CAD build for the part. Positions are in the model's coordinates, mm. Face numbers are marked on the shaded views. A direction names the side the tool comes from. Give positions to 0.01 mm unless a question says otherwise; leave off trailing zeros. Write each loop counter-clockwise with the first axis right and the second up, starting at its lowest first coordinate (ties: lowest second). Pieces come first, ordered by that corner, then holes. Notation, with made-up numbers: (-8, 62.25) -> (9, 62.25) arc R23 ccw to (9, 86.25) -> close; hole circle Ø8 at (17.25, 83). An arc over 180 degrees is marked (long way). Answer as a JSON object with one key per item and string values.
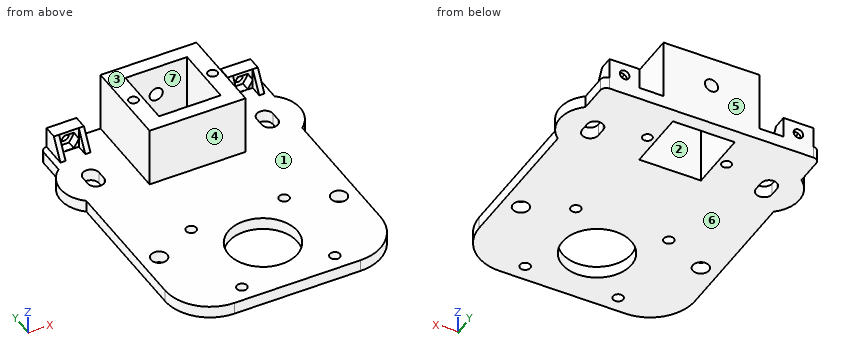
```python
from build123d import *

# Parameters (mm, degrees)
SKETCH_1_R          = 1.7
SKETCH_1_R_2        = 11.5
SKETCH_1_R_3        = 2.7
SKETCH_1_R_4        = 1.6
SKETCH_1_W          = 20.6
SKETCH_1_H          = 20.6
EXTRUDE_1_DEPTH     = 4
EXTRUDE_START       = 4
SKETCH_1_3_W        = 10
SKETCH_1_3_H        = 4.5
EXTRUDE_2_DEPTH     = 7
SKETCH_1_4_W        = 32
SKETCH_1_4_H        = 30
SKETCH_1_4_R        = 1.6
SKETCH_1_4_W_2      = 20.6
SKETCH_1_4_H_2      = 20.6
EXTRUDE_3_DEPTH     = 20
RIB_1_REACH         = 94.748
SKETCH_3_WALL_W     = 195.558888446
SKETCH_3_WALL_H     = 1.7
RIB_2_REACH         = 86.984
SKETCH_4_WALL_W     = 180.029901728
SKETCH_4_WALL_H     = 1.7
CUT_EXTRUDE_1_REACH = 104.259
SKETCH_5_R          = 2.2
SKETCH_5_R_2        = 1.6
CUT_EXTRUDE_2_DEPTH = 3


with BuildPart() as part:
    # 草图1 → 凸台-拉伸1 (new body)
    with BuildSketch(Plane.XY):
        with BuildLine():
            ThreePointArc((36, 48.5), (35.414213562, 49.914213562), (34, 50.5))
            Line((34, 50.5), (-34, 50.5))
            ThreePointArc((-34, 50.5), (-35.414213562, 49.914213562), (-36, 48.5))
            Line((-36, 48.5), (-36, 39.485281374))
            ThreePointArc((-36, 39.485281374), (-40, 31), (-36, 22.514718626))
            Line((-36, 22.514718626), (-36, -25.5))
            ThreePointArc((-36, -25.5), (-31.606601718, -36.106601718), (-21, -40.5))
            Line((-21, -40.5), (21, -40.5))
            ThreePointArc((21, -40.5), (31.606601718, -36.106601718), (36, -25.5))
            Line((36, -25.5), (36, 22.514718626))
            ThreePointArc((36, 22.514718626), (40, 31), (36, 39.485281374))
            Line((36, 39.485281374), (36, 48.5))
        make_face()
        with Locations((-15.5, -35)):
            Circle(SKETCH_1_R, mode=Mode.SUBTRACT)
        with Locations((15.5, -35)):
            Circle(SKETCH_1_R, mode=Mode.SUBTRACT)
        with Locations((0, -19.5)):
            Circle(SKETCH_1_R_2, mode=Mode.SUBTRACT)
        with Locations((-30, -11)):
            Circle(SKETCH_1_R_3, mode=Mode.SUBTRACT)
        with Locations((-15.5, -4)):
            Circle(SKETCH_1_R, mode=Mode.SUBTRACT)
        with Locations((30, -11)):
            Circle(SKETCH_1_R_3, mode=Mode.SUBTRACT)
        with Locations((15.5, -4)):
            Circle(SKETCH_1_R, mode=Mode.SUBTRACT)
        with BuildLine():
            Line((-26.3, 32.5), (-26.3, 29.5))
            ThreePointArc((-26.3, 29.5), (-29, 26.8), (-31.7, 29.5))
            Line((-31.7, 29.5), (-31.7, 32.5))
            ThreePointArc((-31.7, 32.5), (-29, 35.2), (-26.3, 32.5))
        make_face(mode=Mode.SUBTRACT)
        with BuildLine():
            Line((31.7, 32.5), (31.7, 29.5))
            ThreePointArc((31.7, 29.5), (29, 26.8), (26.3, 29.5))
            Line((26.3, 29.5), (26.3, 32.5))
            ThreePointArc((26.3, 32.5), (29, 35.2), (31.7, 32.5))
        make_face(mode=Mode.SUBTRACT)
        with Locations((13.2, 35.5)):
            Circle(SKETCH_1_R_4, mode=Mode.SUBTRACT)
        with Locations((0, 35.5)):
            Rectangle(SKETCH_1_W, SKETCH_1_H, mode=Mode.SUBTRACT)
        with Locations((-13.2, 35.5)):
            Circle(SKETCH_1_R_4, mode=Mode.SUBTRACT)
    extrude(amount=EXTRUDE_1_DEPTH)

    # 草图1<3> → 凸台-拉伸2 (add)
    with BuildSketch(Plane.XY.offset(EXTRUDE_START)):
        with Locations((-29, 48.25)):
            Rectangle(SKETCH_1_3_W, SKETCH_1_3_H)
        with Locations((29, 48.25)):
            Rectangle(SKETCH_1_3_W, SKETCH_1_3_H)
    extrude(amount=EXTRUDE_2_DEPTH)

    # 草图1<4> → 凸台-拉伸3 (add)
    with BuildSketch(Plane.XY.offset(EXTRUDE_START)):
        with Locations((0, 35.5)):
            Rectangle(SKETCH_1_4_W, SKETCH_1_4_H)
        with Locations((-13.2, 35.5)):
            Circle(SKETCH_1_4_R, mode=Mode.SUBTRACT)
        with Locations((0, 35.5)):
            Rectangle(SKETCH_1_4_W_2, SKETCH_1_4_H_2, mode=Mode.SUBTRACT)
        with Locations((13.2, 35.5)):
            Circle(SKETCH_1_4_R, mode=Mode.SUBTRACT)
    extrude(amount=EXTRUDE_3_DEPTH)

    # 草图3 wall → 筋1 (add, up to next)
    with BuildSketch(Plane(origin=(-34, 44, 7.5), x_dir=(0, -0.496138938357, -0.868243142124), z_dir=(0, -0.868243142124, 0.496138938357)), mode=Mode.PRIVATE) as rib_1_sk1:
        with Locations((0, 0.85)):
            Rectangle(SKETCH_3_WALL_W, SKETCH_3_WALL_H)
    rib_1_tool1 = extrude(rib_1_sk1.sketch, amount=-RIB_1_REACH, mode=Mode.PRIVATE) - part.part
    rib_1 = rib_1_tool1.solids().sort_by_distance((-34, 44, 7.5))[0]
    add(rib_1)

    # 草图4 wall → 筋2 (add, up to next)
    with BuildSketch(Plane(origin=(-24, 44, 7.5), x_dir=(0, -0.496138938357, -0.868243142124), z_dir=(0, 0.868243142124, -0.496138938357)), mode=Mode.PRIVATE) as rib_2_sk1:
        with Locations((0, 0.85)):
            Rectangle(SKETCH_4_WALL_W, SKETCH_4_WALL_H)
    rib_2_tool1 = extrude(rib_2_sk1.sketch, amount=RIB_2_REACH, mode=Mode.PRIVATE) - part.part
    rib_2 = rib_2_tool1.solids().sort_by_distance((-24, 44, 7.5))[0]
    add(rib_2)

    # 镜向1: 筋1, 筋2 across plane
    add(rib_1.mirror(Plane(origin=(0, 0, 0), x_dir=(0, 0, 1), z_dir=(1, 0, 0))))
    add(rib_2.mirror(Plane(origin=(0, 0, 0), x_dir=(0, 0, 1), z_dir=(1, 0, 0))))

    # 草图5 → 切除-拉伸1 (cut, up to next)
    with BuildSketch(Plane(origin=(0, 50.5, 0), x_dir=(1, 0, 0), z_dir=(0, 1, 0)), mode=Mode.PRIVATE) as cut_extrude_1_sk1:
        with Locations(Location((0, -14, 0), (0, 0, 270))):
            Circle(SKETCH_5_R)
    cut_extrude_1_tool1 = extrude(cut_extrude_1_sk1.sketch, amount=-CUT_EXTRUDE_1_REACH, mode=Mode.PRIVATE) & part.part
    # 草图5 → 切除-拉伸1 (cut, up to next)
    with BuildSketch(Plane(origin=(0, 50.5, 0), x_dir=(1, 0, 0), z_dir=(0, 1, 0)), mode=Mode.PRIVATE) as cut_extrude_1_sk2:
        with Locations(Location((29, -7, 0), (0, 0, 270))):
            Circle(SKETCH_5_R_2)
    cut_extrude_1_tool2 = extrude(cut_extrude_1_sk2.sketch, amount=-CUT_EXTRUDE_1_REACH, mode=Mode.PRIVATE) & part.part
    # 草图5 → 切除-拉伸1 (cut, up to next)
    with BuildSketch(Plane(origin=(0, 50.5, 0), x_dir=(1, 0, 0), z_dir=(0, 1, 0)), mode=Mode.PRIVATE) as cut_extrude_1_sk3:
        with Locations(Location((-29, -7, 0), (0, 0, 270))):
            Circle(SKETCH_5_R_2)
    cut_extrude_1_tool3 = extrude(cut_extrude_1_sk3.sketch, amount=-CUT_EXTRUDE_1_REACH, mode=Mode.PRIVATE) & part.part
    add(cut_extrude_1_tool1.solids().sort_by_distance((0, 50.5, 14))[0], mode=Mode.SUBTRACT)
    add(cut_extrude_1_tool2.solids().sort_by_distance((29, 50.5, 7))[0], mode=Mode.SUBTRACT)
    add(cut_extrude_1_tool3.solids().sort_by_distance((-29, 50.5, 7))[0], mode=Mode.SUBTRACT)

    # 草图6 → 切除-拉伸2 (cut)
    with BuildSketch(Plane.XZ.offset(-46)):
        Polygon((-27.325684219, 9.9), (-30.674315781, 9.9), (-32.348631561, 7), (-30.674315781, 4.1), (-27.325684219, 4.1), (-25.651368439, 7), align=None)
        Polygon((32.348631561, 7), (30.674315781, 9.9), (27.325684219, 9.9), (25.651368439, 7), (27.325684219, 4.1), (30.674315781, 4.1), align=None)
    extrude(amount=-CUT_EXTRUDE_2_DEPTH, mode=Mode.SUBTRACT)


solid = part.part
```
1) Slice it at A-A (z = 1.5). State how many separate pieces and enclosed holes the cut face has, then the cut area to 3 significant figures.
Model answer:
{"separate pieces": "1", "enclosed holes": "12", "area": "5,530 mm2"}
2) Wall check: probe 1 along X at (y, z) = (28, 7); probe 2 along Y at (x, z) = (10, 3.5); probe 3 along Y at (x, z) = (15.5, 1.5). Give the ranges that are in metal, low to high.
Model answer:
{"probe 1": "x = -16 to -10.3, 10.3 to 16", "probe 2": "y = -40.5 to -25.18, -13.82 to 25.2, 45.8 to 50.5", "probe 3": "y = -40.5 to -36.7, -33.3 to -5.7, -2.3 to 50.5"}
3) Slice it at D-D (z = 14). List the corners of the cut face in (x, y), then the cut area to 3 significant figures.
Model answer:
{"outline": "(-16, 20.5) -> (16, 20.5) -> (16, 50.5) -> (2.2, 50.5) -> (2.2, 45.8) -> (10.3, 45.8) -> (10.3, 25.2) -> (-10.3, 25.2) -> (-10.3, 45.8) -> (-2.2, 45.8) -> (-2.2, 50.5) -> (-16, 50.5) -> close; hole circle Ø3.2 at (-13.2, 35.5); hole circle Ø3.2 at (13.2, 35.5)", "area": "499 mm2"}
4) 3-axis set-ups, long thin cutter, end or side, ignore diameter. For the marked faces 1, 2, 3 and 4: which of +Z, -Z, +X, -X, +Y, -Y reach the whole face in a straight line?
Model answer:
{"face 1": "+Z, -Y", "face 2": "+Z, -Z", "face 3": "+Z, +X, -X, +Y, -Y", "face 4": "+Z, +X, -X, -Y"}
5) Slice it at C-C (y = 31.5). List the corners of the cut face in (x, z), then the cut area to 3 significant figures.
Model answer:
{"outline": "(-39.99, 0) -> (-31.7, 0) -> (-31.7, 4) -> (-39.99, 4) -> close; (-26.3, 0) -> (-10.3, 0) -> (-10.3, 24) -> (-16, 24) -> (-16, 4) -> (-26.3, 4) -> close; (10.3, 0) -> (26.3, 0) -> (26.3, 4) -> (16, 4) -> (16, 24) -> (10.3, 24) -> close; (31.7, 0) -> (39.99, 0) -> (39.99, 4) -> (31.7, 4) -> close", "area": "422 mm2"}
6) Slice it at B-B (y = -19.5). List the corners of the cut face in (x, z).
Model answer:
{"outline": "(-36, 0) -> (-11.5, 0) -> (-11.5, 4) -> (-36, 4) -> close; (11.5, 0) -> (36, 0) -> (36, 4) -> (11.5, 4) -> close"}
7) Pin check, flat tips, straight feed: pin 1 (6 mm diameter, centred on y = 34, z = 16.5, fed in from -X); pin 2 (1.2 mm diameter, centred on y = 44.5, z = 7, fed in from -X); pin 3 (2 mm diameter, centred on y = -1.5, z = 2.5, fed in from -X). Stop position of each tip, or through.
Model answer:
{"pin 1": "stops at x = -16", "pin 2": "stops at x = -34", "pin 3": "stops at x = -36"}
8) Mould opens along Y. For the marked faces 5, 6 and 7 say: released by +Y, released by -Y, zero draft, split by the parting line, or undercut.
Model answer:
{"face 5": "released by +Y", "face 6": "zero draft", "face 7": "undercut"}
